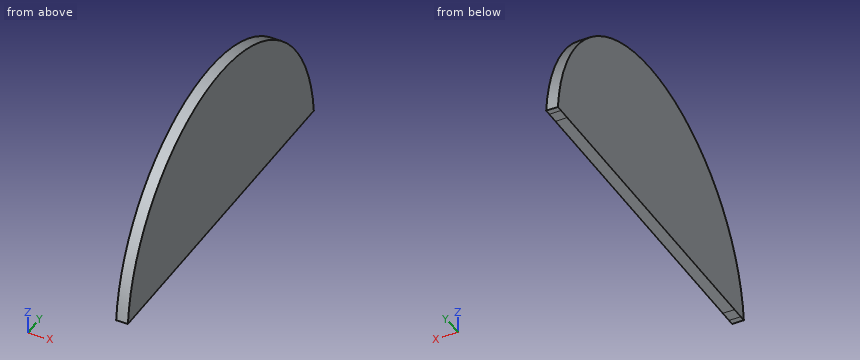
Autodesk Inventor part; units mm, degrees
ref_plane "Work Plane2" through (2.5, -67.5, -250) normal (1, 0, 0) x (0, 1, 0)
ref_plane "Work Plane3" through (-2.5, -72.3, -250) normal (-1, 0, 0) x (0, 0, 1)
ref_plane "YZ Plane" through (0, 0, 0) normal (1, 0, 0) x (0, 1, 0)
ref_plane "Work Plane1" through (-2.5, 0, 34.3925) normal (1, 0, 0) x (0, 1, 0)
sketch "Sketch1" plane through (-2.5, 0, 34.3925) normal (1, 0, 0) x (0, 1, 0)
  arc A0 (72.5, -34.3925) -> (-72.5, -34.3925) centre (0, -45.8883) ccw
  line L0 (72.5, -34.3926) -> (67.5, -34.3926)
  line L1 (67.5, -34.3925) -> (-67.5, -34.3925)
  line L2 (-72.5, -34.3926) -> (-67.5, -34.3926)
  line L3 (67.5, -34.3926) -> (-67.5, -34.3926)
  arc A1 (75, -34.3926) -> (-75, -34.3926) centre (0, -40.8883) ccw
  line L4 (75, -34.3926) -> (-75, -34.3926)
  arc A2 (72.5, -34.3925) -> (-72.5, -34.3925) centre (0, -45.8883) ccw
  line L5 (-72.5, -34.3925) -> (72.5, -34.3925)
  point P0 (0, -34.3925)
  point P1 (-72.5, -34.3926)
  point P2 (72.5, -34.3926)
ref_plane "Work Plane2" through (2.5, -67.5, -250) normal (1, 0, 0) x (0, 1, 0)
ref_plane "Work Plane3" through (-2.5, -72.3, -250) normal (-1, 0, 0) x (0, 0, 1)
extrude "Extrusion1" add sketch "Sketch1" against normal up to surface (5 mm away) from surface at 5
properties part number "Lid2" material "Plastic, Opaque White"
Can you work these out from the model? Positions are in its coordinate system, mm. Coordinates: 2 decimals unless noted, no trailing zeros. Write each loop counter-clockwise with the first axis right and the second up, starting at its lowest first coordinate (ties: lowest second). Pieces come first, ordered by that corner, then holes. Notation, with made-up numbers: (11.25, 19) -> (57.25, 19) arc R16 cw to (57.25, 46) -> close; hole circle Ø1 at (35, 41.5). An arc over 180 degrees is marked (long way). Write each question's results on one line, items separated by ' | '. Start each with the question number.
Q1. I'm going to push flat-ended pins straight in: pin 1 (3 mm diameter, centred on x = -0.5, y = 53.5, fed in from +Z); pin 2 (1.5 mm diameter, centred on x = 0.5, z = 57.5, fed in from -Y). Where does each tip first touch, or does it pass through?
Q2. Imagine slicing it at B-B (y = 42). Write out the boundary of the cut face in (x, z), then the cut area to 3 significant figures.
Q3. Imagine slicing it at C-C (z = 59). Write out the boundary of the cut face in (x, y).
Q4. If I drill on probe 1 along Y at (x, z) = (2.2, 25); probe 2 along Z at (x, y) = (-0.05, -41.5); probe 3 along Z at (x, y) = (-0.9, 23.5), over which ranges is the centre line in solid material (lowest first)?
Q5. Imagine slicing it at A-A (x = 1.2). Write out the boundary of the cut face in (y, z).
Taken from the geometry:
1) pin 1: stops at z = 47.94 | pin 2: stops at y = -40.83
2) outline: (-2.5, 0) -> (2.5, 0) -> (2.5, 55.98) -> (-2.5, 55.98) -> close | area: 280 mm^2
3) outline: (-2.5, -37.11) -> (2.5, -37.11) -> (2.5, 37.11) -> (-2.5, 37.11) -> close
4) probe 1: y = -68.38 to 68.38 | probe 2: z = 0 to 56.31 | probe 3: z = 0 to 65.02
5) outline: (-75, 0) -> (-67.5, 0) -> (67.5, 0) -> (72.5, 0) -> (75, 0) arc R75.28 ccw to start
